Answer from the drawing. Dimensions are ordinates in mm from the lowest x, y and z of the part. A direction names the side the tool comes from. Coordinates: 2 decimals unless noted, no trailing zeros. Order: outer loops, then holes, each group sorted by start corner. A loop starts at its lowest first (then second) coordinate and runs counter-clockwise, first axis right, second up. Notation, with made-up numbers: (39, 2) -> (62, 2) arc R13 cw to (62, 25) -> close; hole circle Ø5 at (43.25, -19.75). An arc over 180 degrees is marked (long way). Answer as a JSON object with one key per item and string values. Group by question number.
1) Consider L1, parallel to X at y = 28, z = 28; L2, parallel to Y at x = 2.5, z = 27; L3, parallel to Y at x = 23, z = 23.5. Determine where each line is inside the solid, lowest interval first.
2) Section C-C on x = 18.5 is taken. Determine the outline of the cut face in (y, z), and give its area (3 significant figures).
3) A tool of negligible diameter and unlimited length cuts with its end or side. For the marked faces 1, 2 and 3, from which of +Z, -Z, +X, -X, +Y, -Y can it reach the whole face along a straight path? Write none if from no direction.
4) Section D-D on y = 19.5 is taken. Determine the outline of the cut face in (x, z).
5) Section B-B on y = 30.5 is taken. Determine the outline of the cut face in (x, z).
6) Section A-A on z = 17 is taken. Determine the outline of the cut face in (x, y).
7) Given pin 1 (6 mm diameter, centred on x = 7, z = 5, fed in from -Y); pin 2 (6 mm diameter, centred on y = 41, z = 7.5, fed in from -X); pin 3 (10 mm diameter, centred on y = 5.5, z = 20.5, fed in from -X); pin 4 (3 mm diameter, centred on y = 16.5, z = 17, fed in from +X), each flat-ended and moving along its own axis, determine where each tip first touches the part or whether it passes through.
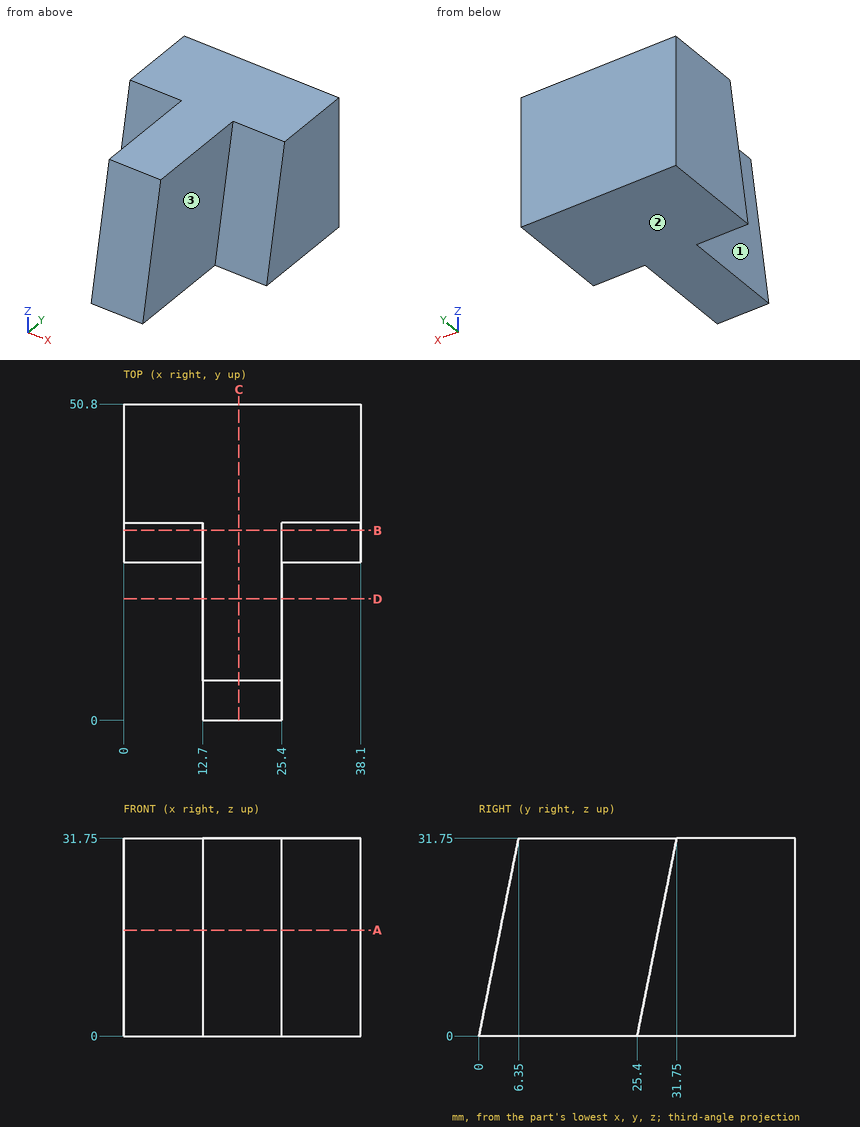
Worked answers:
{
 "1": {"L1": "x = 12.7 to 25.4", "L2": "y = 30.8 to 50.8", "L3": "y = 4.7 to 50.8"},
 "2": {"outline": "(0, 0) -> (50.8, 0) -> (50.8, 31.75) -> (6.35, 31.75) -> close", "area": "1,510 mm²"},
 "3": {"face 1": "+Z, -X, -Y", "face 2": "-Z, +X, -X, +Y, -Y", "face 3": "+Z, +X, -Y"},
 "4": {"outline": "(12.7, 0) -> (25.4, 0) -> (25.4, 31.75) -> (12.7, 31.75) -> close"},
 "5": {"outline": "(0, 0) -> (38.1, 0) -> (38.1, 25.5) -> (25.4, 25.5) -> (25.4, 31.75) -> (12.7, 31.75) -> (12.7, 25.5) -> (0, 25.5) -> close"},
 "6": {"outline": "(0, 28.8) -> (12.7, 28.8) -> (12.7, 3.4) -> (25.4, 3.4) -> (25.4, 28.8) -> (38.1, 28.8) -> (38.1, 50.8) -> (0, 50.8) -> close"},
 "7": {"pin 1": "stops at y = 25.8", "pin 2": "stops at x = 0", "pin 3": "stops at x = 12.7", "pin 4": "stops at x = 25.4"}
}
